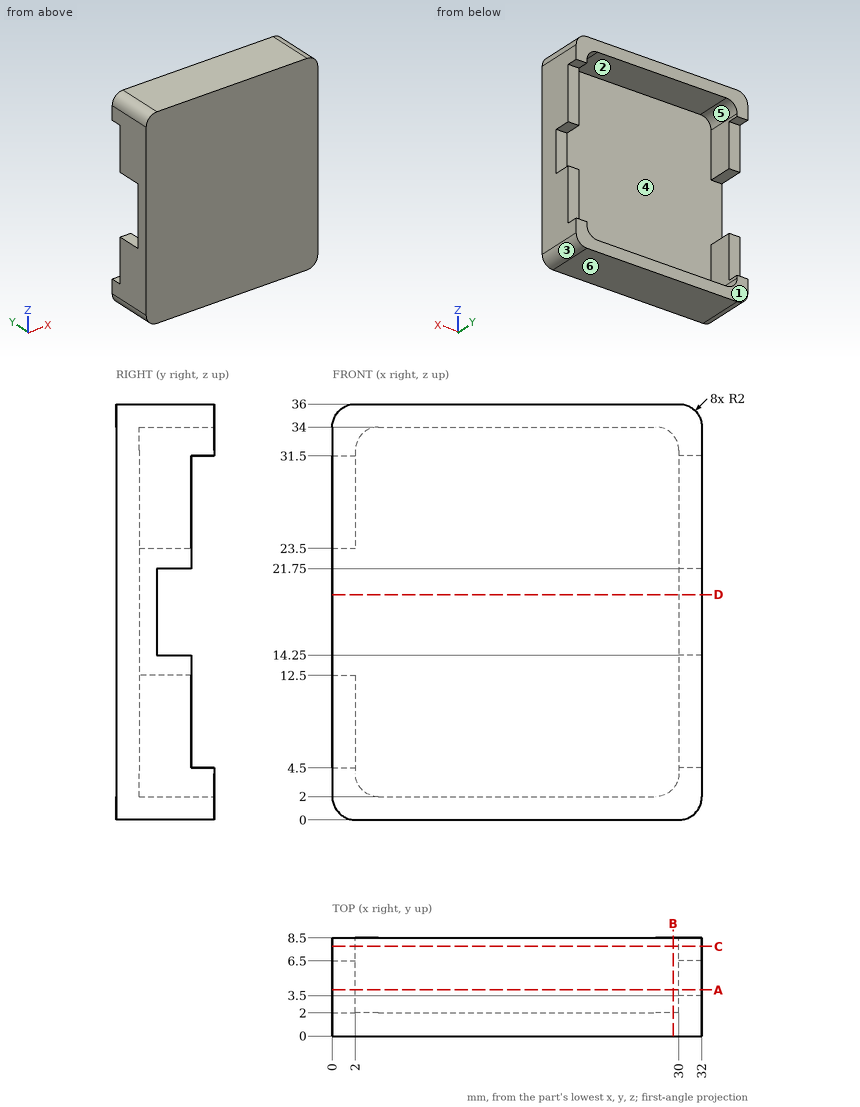
Answer from the drawing. Dimensions are ordinates in mm from the lowest x, y and z of the part. A direction names the side the tool comes from. Give positions to 0.01 mm unless a question says otherwise; leave off trailing zeros. Loops run counter-clockwise (first coordinate to the right, second up) from the corner with the lowest first, then second, coordinate; pieces in that order, holes last. Notation, with made-up numbers: (-32.75, 0) -> (-11.75, 0) arc R24 ccw to (-11.75, 37) -> close; hole circle Ø7 at (43, 12.25). An arc over 180 degrees is marked (long way). One line per question, with ' | ' between items. Start each with the question number.
1) Section C-C, the plane y = 7.75 is taken. Determine the outline of the cut face in (x, z).
2) Section B-B, the plane x = 29.5 is taken. Determine the outline of the cut face in (y, z).
3) Section A-A, the plane y = 4 is taken. Determine the outline of the cut face in (x, z), then the cut area to 3 significant figures.
4) Section D-D, the plane z = 19.5 is taken. Determine the outline of the cut face in (x, y), then the cut area to 3 significant figures.
5) Determine the mould class of the marked faces 1, 2, 3 and 4 for opening direction X: +X half, -X half, draft (parallel to the pull), parting line (faces both ways), or undercut.
6) For the marked faces 5 and 6, determine the directions among +Z, -Z, +X, -X, +Y, -Y from which every point of the face is accessible in a straight line to the end or side of a thin tool.
7) Straight lines are drawn through the part: L1, parallel to Z at x = 18, y = 3.25; L2, parallel to Y at x = 15, z = 27; L3, parallel to X at y = 3.25, z = 4. For each, find the intervals that lie inside material, in ascending order.
8) Each of these flat-tipped pins is pushed along its axis until it touches: pin 1 (1 mm diameter, centred on x = 1.5, z = 26, fed in from +Y); pin 2 (12 mm diameter, centred on x = 13.5, z = 10, fed in from +Y); pin 3 (0.6 mm diameter, centred on x = 1.5, y = 7.5, fed in from +Z); pin 4 (1 mm diameter, centred on y = 7, z = 21, fed in from -X). Where does it stop, or does it pass through?
Resolved:
1) outline: (0, 2) arc R2 ccw to (2, 0) -> (30, 0) arc R2 ccw to (32, 2) -> (32, 4.5) -> (30, 4.5) -> (30, 4) arc R2 cw to (28, 2) -> (4, 2) arc R2 cw to (2, 4) -> (2, 4.5) -> (0, 4.5) -> close; (0, 31.5) -> (2, 31.5) -> (2, 32) arc R2 cw to (4, 34) -> (28, 34) arc R2 cw to (30, 32) -> (30, 31.5) -> (32, 31.5) -> (32, 34) arc R2 ccw to (30, 36) -> (2, 36) arc R2 ccw to (0, 34) -> close
2) outline: (0, 0) -> (8.5, 0) -> (8.5, 2.68) -> (2, 2.68) -> (2, 33.32) -> (8.5, 33.32) -> (8.5, 36) -> (0, 36) -> close
3) outline: (0, 2) arc R2 ccw to (2, 0) -> (30, 0) arc R2 ccw to (32, 2) -> (32, 14.25) -> (30, 14.25) -> (30, 4) arc R2 cw to (28, 2) -> (4, 2) arc R2 cw to (2, 4) -> (2, 12.5) -> (0, 12.5) -> close; (0, 23.5) -> (2, 23.5) -> (2, 32) arc R2 cw to (4, 34) -> (28, 34) arc R2 cw to (30, 32) -> (30, 21.75) -> (32, 21.75) -> (32, 34) arc R2 ccw to (30, 36) -> (2, 36) arc R2 ccw to (0, 34) -> close | area: 219 mm2
4) outline: (0, 0) -> (32, 0) -> (32, 3.5) -> (30, 3.5) -> (30, 2) -> (0, 2) -> close | area: 67.0 mm2
5) face 1: draft | face 2: undercut | face 3: +X half | face 4: undercut
6) face 5: +Y | face 6: -Z, +X, -X, +Y, -Y
7) L1: 0 to 2, 34 to 36 | L2: 0 to 2 | L3: 0 to 2, 30 to 32
8) pin 1: y = 6.5 | pin 2: y = 2 | pin 3: z = 35.99 | pin 4: through
